The listing builds one solid part. Answer for the finished solid, in the listing's coordinates (mm). Face numbers are marked on the shaded views. A direction names the side the tool comes from. Coordinates: 2 decimals unless noted, no trailing zeros. Order: outer loops, then holes, each group sorted by start corner. A loop starts at its lowest first (then second) coordinate and runs counter-clockwise, first axis right, second up. Notation, with made-up numbers: (74, 80) -> (90, 80) arc R19 ccw to (90, 84) -> close; hole circle Ø3 at (-13.75, -4.75). An arc over 180 degrees is marked (long way). Answer in a Markdown table with one row per item. Add a question column.
```python
from build123d import *

# Parameters (mm, degrees)
BOSS_EXTRUDE1_DEPTH = 3
FILLET1_R           = 0.5


with BuildPart() as part:
    # Sketch1 → Boss-Extrude1 (new body)
    with BuildSketch(Plane.XY):
        with BuildLine():
            Line((-5.350435009, -2.26924573), (10.729564991, -2.26924573))
            Line((10.729564991, -2.26924573), (10.729564991, 3.73075427))
            Line((10.729564991, 3.73075427), (7.729564991, 3.73075427))
            Line((7.729564991, 3.73075427), (7.729564991, 2.73075427))
            ThreePointArc((7.729564991, 2.73075427), (7.529564991, 2.23075427), (7.729564991, 1.73075427))
            Line((7.729564991, 1.73075427), (7.729564991, 0.73075427))
            Line((7.729564991, 0.73075427), (4.229564991, 0.73075427))
            Line((4.229564991, 0.73075427), (4.229564991, 5.73075427))
            Line((4.229564991, 5.73075427), (1.149564991, 5.73075427))
            Line((1.149564991, 5.73075427), (1.149564991, 0.73075427))
            Line((1.149564991, 0.73075427), (-2.350435009, 0.73075427))
            Line((-2.350435009, 0.73075427), (-2.350435009, 1.73075427))
            ThreePointArc((-2.350435009, 1.73075427), (-2.150435009, 2.23075427), (-2.350435009, 2.73075427))
            Line((-2.350435009, 2.73075427), (-2.350435009, 3.73075427))
            Line((-2.350435009, 3.73075427), (-5.350435009, 3.73075427))
            Line((-5.350435009, 3.73075427), (-5.350435009, -2.26924573))
        make_face()
    extrude(amount=BOSS_EXTRUDE1_DEPTH)

    # Fillet1
    fillet1_edges = [part.edges().sort_by_distance(p)[0] for p in [
        (-2.350435009, 3.73075427, 1.5),
        (7.729564991, 3.73075427, 1.5),
    ]]
    fillet(fillet1_edges, radius=FILLET1_R)


solid = part.part
```
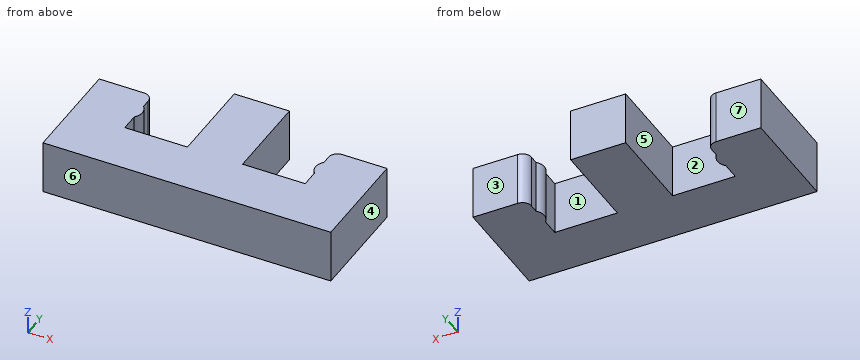
Q1. A cutting plane is placed at D-D (y = 4.75). Determine the outline of the cut face in (x, z).
Q2. Given pin 1 (1.5 mm diameter, centred on x = -1, z = 1.5, fed in from +Y); pin 2 (0.8 mm diameter, centred on x = -4, z = 1.5, fed in from +Y), each flat-ended and moving along its own axis, determine where each tip first touches the part or whether it passes through.
Q3. Straight lines are drawn through the part: line 1 (X direction, y = 1.25, z = 2.2); line 2 (X direction, y = 2.25, z = 2.4); line 3 (Y direction, x = 9.25, z = 2.05). For each, find the intervals that lie inside material, in ascending order.
Q4. A cutting plane is placed at C-C (x = 8.75). Determine the outline of the cut face in (y, z).
Q5. A cutting plane is placed at B-B (z = 1.65). Determine the outline of the cut face in (x, y) (3 decimals).
Q6. For the marked faces 5, 6 and 7, determine the directions among +Z, -Z, +X, -X, +Y, -Y from which every point of the face is accessible in a straight line to the end or side of a thin tool.
Q7. Determine the mould class of the marked faces 1, 2, 3 and 4 for opening direction X: +X half, -X half, draft (parallel to the pull), parting line (faces both ways), or undercut.
Q8. A cutting plane is placed at A-A (y = 1.5). Determine the outline of the cut face in (x, z).
Returned:
| question | item | result |
|---|---|---|
| 1 | outline | (1.15, 0) -> (4.23, 0) -> (4.23, 3) -> (1.15, 3) -> close |
| 2 | pin 1 | stops at y = 0.73 |
| 2 | pin 2 | stops at y = 3.73 |
| 3 | line 1 | x = -5.35 to -2.35, 1.15 to 4.23, 7.73 to 10.73 |
| 3 | line 2 | x = -5.35 to -2.15, 1.15 to 4.23, 7.53 to 10.73 |
| 3 | line 3 | y = -2.27 to 3.73 |
| 4 | outline | (-2.27, 0) -> (3.73, 0) -> (3.73, 3) -> (-2.27, 3) -> close |
| 5 | outline | (-5.35, -2.269) -> (10.73, -2.269) -> (10.73, 3.731) -> (8.23, 3.731) arc R0.5 ccw to (7.73, 3.231) -> (7.73, 2.731) arc R0.725 ccw to (7.73, 1.731) -> (7.73, 0.731) -> (4.23, 0.731) -> (4.23, 5.731) -> (1.15, 5.731) -> (1.15, 0.731) -> (-2.35, 0.731) -> (-2.35, 1.731) arc R0.725 ccw to (-2.35, 2.731) -> (-2.35, 3.231) arc R0.5 ccw to (-2.85, 3.731) -> (-5.35, 3.731) -> close |
| 6 | face 5 | +Z, -Z, +Y |
| 6 | face 6 | +Z, -Z, +X, -X, -Y |
| 6 | face 7 | +Z, -Z, -X, +Y |
| 7 | face 1 | undercut |
| 7 | face 2 | undercut |
| 7 | face 3 | draft |
| 7 | face 4 | +X half |
| 8 | outline | (-5.35, 0) -> (-2.35, 0) -> (-2.35, 3) -> (-5.35, 3) -> close; (1.15, 0) -> (4.23, 0) -> (4.23, 3) -> (1.15, 3) -> close; (7.73, 0) -> (10.73, 0) -> (10.73, 3) -> (7.73, 3) -> close |
